from build123d import *

# Parameters (mm, degrees)
CROQUIS1_R              = 25
CROQUIS1_R_2            = 2
SALIENTE_EXTRUIR1_DEPTH = 20
SALIENTE_EXTRUIR2_DEPTH = 10
SALIENTE_EXTRUIR3_DEPTH = 12.5
CROQUIS5_W              = 20
CROQUIS5_H              = 20
CORTAR_EXTRUIR1_DEPTH   = 10
CROQUIS6_R              = 2
CORTAR_EXTRUIR2_DEPTH   = 10
CROQUIS7_R              = 2
CORTAR_EXTRUIR3_DEPTH   = 143.653426177
CORTAR_EXTRUIR4_DEPTH   = 5
REDONDEO1_R             = 25
SALIENTE_EXTRUIR4_DEPTH = 10
CORTAR_EXTRUIR5_DEPTH   = 10


with BuildPart() as part:
    # Croquis1 → Saliente-Extruir1 (new body)
    with BuildSketch(Plane(origin=(0, 0, 0), x_dir=(1, 0, 0), z_dir=(0, 1, 0))):
        with Locations(Location((0, 0, 0), (0, 0, 270))):
            Circle(CROQUIS1_R)
        with Locations(Location((0, 0, 0), (0, 0, 270))):
            Circle(CROQUIS1_R_2, mode=Mode.SUBTRACT)
    extrude(amount=SALIENTE_EXTRUIR1_DEPTH)

    # Croquis3 → Saliente-Extruir2 (add, symmetric)
    with BuildSketch(Plane(origin=(0, 0, 0), x_dir=(0, 0, -1), z_dir=(1, 0, 0))):
        Polygon((0, 20), (25, 16), (87.155173578, 6.055172228), (105, -40.652023899), (105, -70), (85, -70), (85, -44.34250964), (72.489864787, -11.598378366), (25, -4), (0, 0), align=None)
    extrude(amount=SALIENTE_EXTRUIR2_DEPTH, both=True)

    # Croquis4 → Saliente-Extruir3 (add)
    with BuildSketch(Plane(origin=(0, 0, 0), x_dir=(1, 0, 0), z_dir=(0, -0.9874406319167053, 0.15799050110667304))):
        with BuildLine():
            Line((-10, -48.018489352), (-29.097101252, -19.451444643))
            ThreePointArc((-29.097101252, -19.451444643), (0, 35), (29.097101252, -19.451444643))
            Line((29.097101252, -19.451444643), (10, -48.018489352))
            Line((10, -48.018489352), (-10, -48.018489352))
        make_face()
    extrude(amount=-SALIENTE_EXTRUIR3_DEPTH)

    # Croquis5 → Cortar-Extruir1 (cut)
    with BuildSketch(Plane(origin=(10, 0, 0), x_dir=(0, 0, -1), z_dir=(1, 0, 0))):
        with Locations((95, -60)):
            Rectangle(CROQUIS5_W, CROQUIS5_H)
    extrude(amount=-CORTAR_EXTRUIR1_DEPTH, mode=Mode.SUBTRACT)

    # Croquis6 → Cortar-Extruir2 (cut)
    with BuildSketch(Plane(origin=(0, 0, 0), x_dir=(0, 0, -1), z_dir=(1, 0, 0))):
        with Locations((100, -55)):
            Circle(CROQUIS6_R)
        with Locations((100, -65)):
            Circle(CROQUIS6_R)
        with Locations((90, -65)):
            Circle(CROQUIS6_R)
        with Locations((90, -55)):
            Circle(CROQUIS6_R)
    extrude(amount=-CORTAR_EXTRUIR2_DEPTH, mode=Mode.SUBTRACT)

    # Croquis7 → Cortar-Extruir3 (cut, through all)
    with BuildSketch(Plane(origin=(0, 20, 0), x_dir=(1, 0, 0), z_dir=(0, 1, 0))):
        with Locations(Location((0, 0, 0), (0, 0, 180))):
            Circle(CROQUIS7_R)
    extrude(amount=-CORTAR_EXTRUIR3_DEPTH, mode=Mode.SUBTRACT)

    # Croquis8 → Cortar-Extruir4 (cut, symmetric)
    with BuildSketch(Plane.XZ):
        Polygon((5, 0), (2.5, 4.330127019), (-2.5, 4.330127019), (-5, 0), (-2.5, -4.330127019), (2.5, -4.330127019), align=None)
    extrude(amount=CORTAR_EXTRUIR4_DEPTH, both=True, mode=Mode.SUBTRACT)

    # Redondeo1
    redondeo1_edges = [part.edges().sort_by_distance(p)[0] for p in [
        (0, -11.598378366, -72.489864787),
        (0, -44.34250964, -85),
        (0, -40.652023899, -105),
        (0, 6.055172228, -87.155173578),
    ]]
    fillet(redondeo1_edges, radius=REDONDEO1_R)

    # Croquis9 → Saliente-Extruir4 (add)
    with BuildSketch(Plane.ZY.offset(10)):
        with BuildLine():
            Line((-85, -70), (-84.332978708, -70))
            ThreePointArc((-84.332978708, -70), (-84.831826004, -68.238225633), (-85, -66.414927782))
            Line((-85, -66.414927782), (-85, -70))
        make_face()
    extrude(amount=-SALIENTE_EXTRUIR4_DEPTH)

    # Croquis10 → Cortar-Extruir5 (cut)
    with BuildSketch(Plane(origin=(0, 0, 0), x_dir=(0, 0, -1), z_dir=(1, 0, 0))):
        Polygon((105, -66.754605318), (105, -70), (104.45872155, -70), (104.782079233, -68.830882246), align=None)
    extrude(amount=-CORTAR_EXTRUIR5_DEPTH, mode=Mode.SUBTRACT)


solid = part.part
Here's how the part is built. I have some questions about the finished solid (model axes, mm). A direction names the side the tool comes from. Coordinates: 2 decimals unless noted, no trailing zeros. Order: outer loops, then holes, each group sorted by start corner. A loop starts at its lowest first (then second) coordinate and runs counter-clockwise, first axis right, second up.
Item 1: If we section it at C-C on z = -51: List the corners of the cut face in (x, y) for me, plus the area to 3 significant figures.
Result sheet:
outline: (-10, -8.16) - (10, -8.16) - (10, 11.84) - (-10, 11.84) - close
area: 400 mm2
Item 2: I need wall thicknesses on line 1 (Y direction, x = -5.25, z = -90); line 2 (X direction, y = 6.5, z = -60); line 3 (Y direction, x = -14, z = 4). Which ranges of each line are inside material? Lowest first, please.
Result sheet:
line 1: y = -70 to -67, -63 to -57, -53 to -2.86
line 2: x = -10 to 10
line 3: y = 0 to 20
Item 3: For P1, Ø4, axis at x = -1, y = 2, coming from the -Z side; P2, Ø5, axis at x = -6.5, z = -51.5, coming from the +Y side; P3, Ø2, axis at x = 5, y = -33.5, coming from the +Z side, each with a flat end and sliding along its axis, tell me the tip position at first contact or that it passes through.
Result sheet:
P1: stops at z = -87.86
P2: stops at y = 12.16
P3: stops at z = -80.48
Item 4: If we mould it in two halves opening along Z, with no side actions, what happens to faces 5 (the face through (0, -60, -95)), 6 (the face through (-0.14, -40.666, -104.573)), 7 (the face through (-3.77, 2.11, -2.13))? For each: +Z half, -Z half, draft (parallel to the pull), parting line (faces both ways), or undercut.
Result sheet:
face 5: draft
face 6: -Z half
face 7: undercut
Item 5: For faces 1 (the face through (-15.39, 9.4, -20.36)), 2 (the face through (0, 0, 10)), 3 (the face through (3.73, 2.11, -2.2)), 4 (the face through (-7, -58, -85)), which set-ups out of +Z, -Z, +X, -X, +Y, -Y let a thin tool reach every point of the face, with its end or its side?
Result sheet:
face 1: +Y
face 2: +Z, +X, -X, -Y
face 3: -Y
face 4: +Z, +X, -X
Item 6: If we section it at D-D on y = -30.5: List the corners of the cut face in (x, z) for me.
Result sheet:
outline: (-10, -101.12) - (10, -101.12) - (10, -79.71) - (-10, -79.71) - close
Item 7: If we section it at A-A on z = -100: List the corners of the cut face in (x, y) for me.
Result sheet:
outline: (-10, -70) - (0, -70) - (0, -67) - (-10, -67) - close; (-10, -63) - (0, -63) - (0, -57) - (-10, -57) - close; (-10, -53) - (0, -53) - (0, -50) - (10, -50) - (10, -27.56) - (-10, -27.56) - close
Item 8: If we section it at B-B on x = -15: List the corners of the cut face in (y, z) for me, plus the area to 3 significant figures.
Result sheet:
outline: (-6.4, -40.03) - (5.94, -42) - (9.46, -20) - (20, -20) - (20, 20) - (15.86, 20) - (17.34, 29.25) - (5, 31.23) - (3.2, 20) - (0, 20) - (0, 0) - close
area: 1,230 mm2
